Work out the finished part from the listing and answer in its coordinate system (mm). A direction names the side the tool comes from. Round coordinates to 2 decimals unless told otherwise and drop trailing zeros. Write each loop counter-clockwise with the first axis right and the second up, starting at its lowest first coordinate (ties: lowest second). Pieces come first, ordered by that corner, then holes. Notation, with made-up numbers: M 37.25,64.25 L 61.25,64.25 A18 ccw 61.25,90.25 Z; hole C 89,33 d2. An arc over 180 degrees is marked long. One line per item, written item: value. Start each with the question number.
Q1. Find section A-A (x = 0). Write down the section's boundary in (y, z).
Q2. Find section B-B (z = 0). Write down the section's boundary in (x, y), and give its area (3 significant figures).
Q3. The mould has two halves that part along X. Classify faces 3 (the cylindrical face through (15.9, 49.2, 1.2)), 4 (the flat face through (0, 78.7, 0)), 5 (the cylindrical face through (-1.08, 66.03, -4.88)), 6 (the cylindrical face through (-0.26, 49.235, 15.517)): released by +X, released by -X, zero draft, split by the parting line, or undercut.
Q4. Consider probe 1 along Y at (x, z) = (13, -10); probe 2 along Z at (x, y) = (17, 48); probe 3 along Y at (x, z) = (11, 1.5). Determine where each line is inside the solid, lowest interval first.
Q5. Given pin 1 Ø3 at (x, z) = (18, -1) entering from +Y; pin 2 Ø2 at (x, z) = (-0.5, -18) entering from +Y; pin 3 Ø5 at (x, y) = (6.5, 51) entering from +Z, each flat-ended and moving along its own axis, determine where each tip first touches the part or whether it passes through.
Q6. A tool of negligible diameter and unlimited length cuts with its end or side. For faces 1 (the flat face through (0, 0, 0)), 2 (the flat face through (6, 53.7, 0)), from which of +Z, -Z, +X, -X, +Y, -Y can it reach the whole face along a straight path? Write none if from no direction.
Q7. Find section C-C (y = 18). Write down the section's boundary in (x, z), and give its area (3 significant figures).
Q8. Find section D-D (z = 11.5). Write down the section's boundary in (x, y), and give its area (3 significant figures).
Autodesk Inventor part; units mm, degrees
ref_plane "YZ Plane" through (0, 0, 0) normal (1, 0, 0) x (0, 1, 0)
ref_plane "XZ Plane" through (0, 0, 0) normal (0, 1, 0) x (-1, 0, 0)
ref_plane "XY Plane" through (0, 0, 0) normal (0, 0, 1) x (1, 0, 0)
sketch "Sketch1" plane through (0, 0, 0) normal (0, 1, 0) x (-1, 0, 0)
  circle A0 centre (0, 0) radius 21
  dimension "d0" = 42
extrude "Extrusion1" add sketch "Sketch1" along normal blind 51.7
sketch "Sketch2" plane through (0, 51.7, 0) normal (0, 1, 0) x (1, 0, 0)
  circle A0 centre (0, 0) radius 13
  dimension "d3" = 26
extrude "Extrusion2" add sketch "Sketch2" along normal blind 2
sketch "Sketch3" plane through (0, 53.7, 0) normal (0, 1, 0) x (1, 0, 0)
  circle A0 centre (0, 0) radius 5
  dimension "d6" = 10
extrude "Extrusion3" add sketch "Sketch3" along normal blind 25
sketch "Sketch4" plane through (0, 51.7, 0) normal (0, 1, 0) x (1, 0, 0)
  circle A0 centre (0, -17.5) radius 2
  line L0 (0, -17.5) -> (0, 0) construction
  circle A1 centre (17.5, 0) radius 2
  circle A2 centre (0, 17.5) radius 2
  circle A3 centre (-17.5, 0) radius 2
  dimension "d9" = 4
  dimension "d10" = 17.5
  dimension "d13" = 360
extrude "Extrusion4" cut sketch "Sketch4" against normal blind 5
properties part number "27-1 Gearbox" material "Aluminum 6061"
The answers:
1. outline: M 0,-21 L 51.7,-21 L 51.7,-19.5 L 46.7,-19.5 L 46.7,-15.5 L 51.7,-15.5 L 51.7,-13 L 53.7,-13 L 53.7,-5 L 78.7,-5 L 78.7,5 L 53.7,5 L 53.7,13 L 51.7,13 L 51.7,15.5 L 46.7,15.5 L 46.7,19.5 L 51.7,19.5 L 51.7,21 L 0,21 Z
2. outline: M -21,0 L 21,0 L 21,51.7 L 19.5,51.7 L 19.5,46.7 L 15.5,46.7 L 15.5,51.7 L 13,51.7 L 13,53.7 L 5,53.7 L 5,78.7 L -5,78.7 L -5,53.7 L -13,53.7 L -13,51.7 L -15.5,51.7 L -15.5,46.7 L -19.5,46.7 L -19.5,51.7 L -21,51.7 Z
2. area: 2,430 mm2
3. face 3: undercut
3. face 4: zero draft
3. face 5: split by the parting line
3. face 6: undercut
4. probe 1: 0 to 51.7
4. probe 2: -12.33 to -1.94, 1.94 to 12.33
4. probe 3: 0 to 53.7
5. pin 1: y = 51.7
5. pin 2: y = 46.7
5. pin 3: z = 20.62
6. face 1: +Z, -Z, +X, -X, -Y
6. face 2: +Y
7. outline: C 0,0 d42
7. area: 1,390 mm2
8. outline: M -17.57,0 L 17.57,0 L 17.57,51.7 L 6.06,51.7 L 6.06,53.7 L -6.06,53.7 L -6.06,51.7 L -17.57,51.7 Z
8. area: 1,840 mm2
